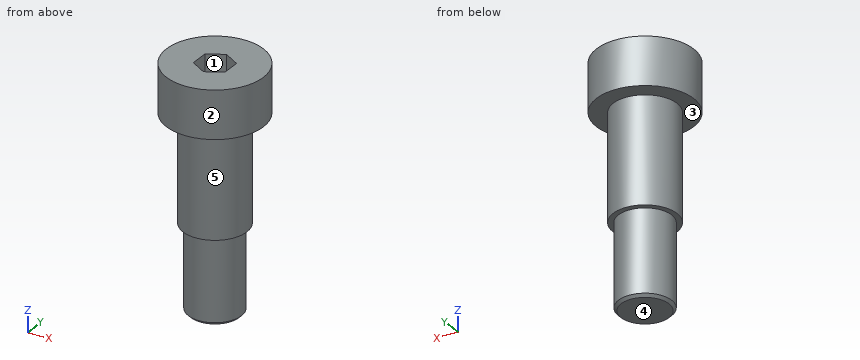
Solid Edge part; units mm, degrees
sketch "Sketch1" plane through (0, 0, 0) normal (0, 0, 1) x (1, 0, 0)
  circle A0 centre (0, 0) radius 9.135
extrude "Protrusion1" add sketch "Sketch1" along normal blind 9
sketch "Sketch2" plane through (0, 0, 9) normal (0, 0, 1) x (1, 0, 0)
  line L0 (0, -3.4641) -> (-3, -1.7321)
  line L1 (-3, -1.7321) -> (-3, 1.7321)
  line L2 (-3, 1.7321) -> (0, 3.4641)
  line L3 (0, 3.4641) -> (3, 1.7321)
  line L4 (3, 1.7321) -> (3, -1.7321)
  line L5 (3, -1.7321) -> (0, -3.4641)
extrude "Cutout1" cut sketch "Sketch2" against normal blind 4.5
sketch "Sketch3" plane through (0, 0, 0) normal (0, 0, -1) x (0, 1, 0)
  circle A0 centre (0, 0) radius 6
extrude "Protrusion2" add sketch "Sketch3" along normal blind 20
sketch "Sketch4" plane through (0, 0, -20) normal (0, 0, -1) x (0, 1, 0)
  circle A0 centre (0, 0) radius 5
extrude "Protrusion3" add sketch "Sketch4" along normal blind 16
chamfer "Chamfer1" distance 0.5 angle 45 1 edges at (0, -5, -36)
properties part number "113690"
For this review, take the finished solid that the model builds, in its own axes (mm). Face numbers are marked on the shaded views. A direction names the side the tool comes from. Coordinates: 2 decimals unless noted, no trailing zeros. Write each loop counter-clockwise with the first axis right and the second up, starting at its lowest first coordinate (ties: lowest second). Pieces come first, ordered by that corner, then holes.
(1) Tool access review of the marked faces 4 and 5: name each direction out of +Z, -Z, +X, -X, +Y, -Y from which nothing blocks a thin tool from reaching the whole face with its end or side.
(2) Add section B-B on z = 4. Give the boundary of the cut face in (x, y) (3 decimals).
(3) Wall thickness on probe 1 along X at (y, z) = (-0.25, -21.5); probe 2 along Z at (x, y) = (1.5, -6.25); probe 3 along Z at (x, y) = (1.5, -2.5): over which ranges is each line inside the solid? List them lowest first.
(4) Add section A-A on y = 0. Give the boundary of the cut face in (x, z) (3 decimals).
(5) The part is to be moulded in two halves that separate along Y. For the marked faces 1, 2 and 3, say which applies: +Y half, -Y half, draft (parallel to the pull), parting line (faces both ways), or undercut.
(6) Add section C-C on x = -7.5. Give the boundary of the cut face in (y, z).
(7) For pin 1 Ø5 at (x, y) = (-0.5, -1.5) entering from +Z; pin 2 Ø6 at (y, z) = (-7, -28.5) entering from -X; pin 3 Ø3 at (x, z) = (-6, -29.5) entering from +Y; pin 4 Ø2 at (x, z) = (5.5, 3.5) entering from +Y, all flat-tipped, find the tip position at first contact; note any pin that passes through.
(8) Add section D-D on z = -11. Give the boundary of the cut face in (x, y), then the cut area to 3 significant figures.
Answer sheet:
1. face 4: -Z, +X, -X, +Y, -Y
1. face 5: -Z
2. outline: circle Ø18.27 at (0, 0)
3. probe 1: x = -4.99 to 4.99
3. probe 2: z = 0 to 9
3. probe 3: z = -36 to 4.5
4. outline: (-9.135, 0) - (-6, 0) - (-6, -20) - (-5, -20) - (-5, -35.5) - (-4.5, -36) - (4.5, -36) - (5, -35.5) - (5, -20) - (6, -20) - (6, 0) - (9.135, 0) - (9.135, 9) - (3, 9) - (3, 4.5) - (-3, 4.5) - (-3, 9) - (-9.135, 9) - close
5. face 1: undercut
5. face 2: parting line
5. face 3: draft
6. outline: (-5.22, 0) - (5.22, 0) - (5.22, 9) - (-5.22, 9) - close
7. pin 1: stops at z = 9
7. pin 2: stops at x = -3
7. pin 3: stops at y = 2.18
7. pin 4: stops at y = 7.95
8. outline: circle Ø12 at (0, 0)
8. area: 113 mm2
